Part print with two shaded views. Sizes in mm from the minimum x, y, z corner. Round coordinates to 2 decimals unless told otherwise and drop trailing zeros. Order: outer loops, then holes, each group sorted by start corner. A loop starts at its lowest first (then second) coordinate and runs counter-clockwise, first axis right, second up. Notation, with made-up numbers: M 84,37.5 L 116,37.5 A12 ccw 116,59.5 Z; hole C 54,66.5 d7. An arc over 180 degrees is marked long. One line per question, with ' | ' between items.
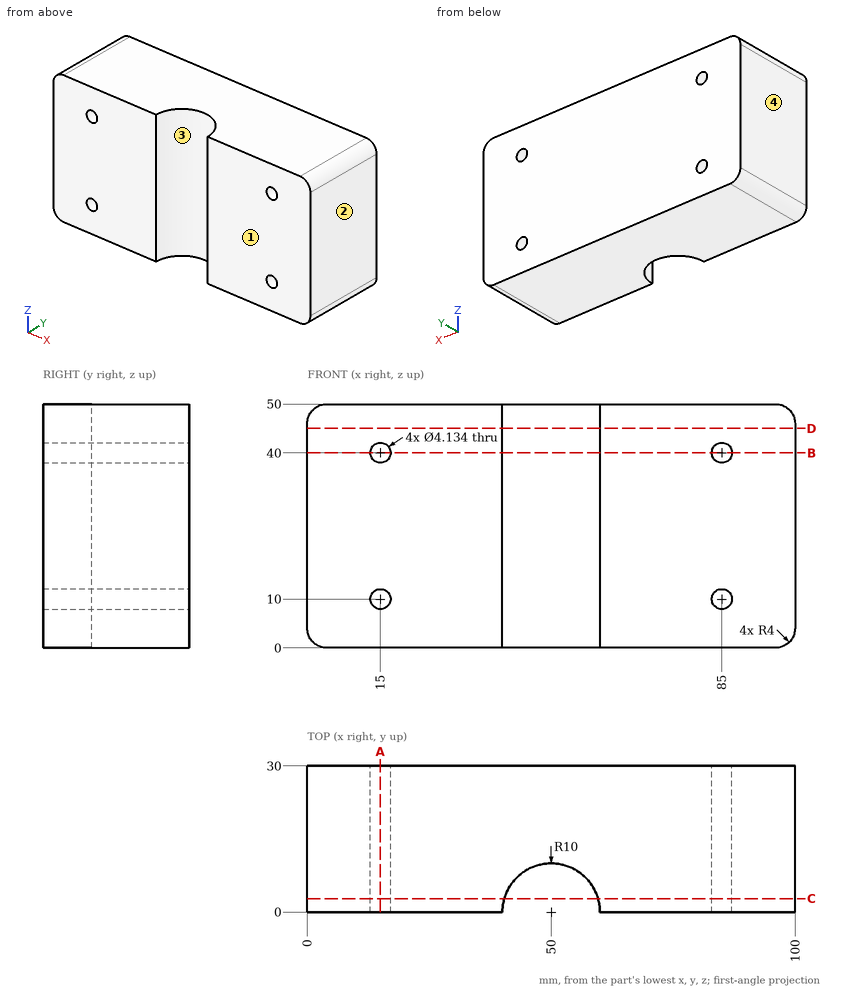
1) Saw through at D-D (z = 45). List the corners of the cut face in (x, y), plus the area to 3 significant figures.
The answers:
outline: M 0,0 L 40,0 A10 cw 60,0 L 100,0 L 100,30 L 0,30 Z | area: 2,840 mm²
2) Probe line 1 (Z direction, x = 15, y = 19.5); line 2 (X direction, y = 15, z = 10); line 3 (X direction, y = 7.5, z = 10). List the from-to ranges inside material, lowest first. Write a range as [from, to].
The answers:
line 1: z = [0, 7.93], [12.07, 37.93], [42.07, 50] | line 2: x = [0, 12.93], [17.07, 82.93], [87.07, 100] | line 3: x = [0, 12.93], [17.07, 43.39], [56.61, 82.93], [87.07, 100]
3) Saw through at B-B (z = 40). List the corners of the cut face in (x, y).
The answers:
outline: M 0,0 L 12.93,0 L 12.93,30 L 0,30 Z; M 17.07,0 L 40,0 A10 cw 60,0 L 82.93,0 L 82.93,30 L 17.07,30 Z; M 87.07,0 L 100,0 L 100,30 L 87.07,30 Z
4) Saw through at C-C (y = 2.75). List the corners of the cut face in (x, z).
The answers:
outline: M 0,4 A4 ccw 4,0 L 40.39,0 L 40.39,50 L 4,50 A4 ccw 0,46 Z; M 59.61,0 L 96,0 A4 ccw 100,4 L 100,46 A4 ccw 96,50 L 59.61,50 Z; hole C 15,10 d4.13; hole C 15,40 d4.13; hole C 85,10 d4.13; hole C 85,40 d4.13
5) Two-plate mould, pull along X, no slides. Class the marked faces 1, 2, 3 and 4: released by +X, released by -X, zero draft, split by the parting line, or undercut.
The answers:
face 1: zero draft | face 2: released by +X | face 3: undercut | face 4: released by -X
6) Saw through at A-A (x = 15). List the corners of the cut face in (y, z), plus the area to 3 significant figures.
The answers:
outline: M 0,0 L 30,0 L 30,7.93 L 0,7.93 Z; M 0,12.07 L 30,12.07 L 30,37.93 L 0,37.93 Z; M 0,42.07 L 30,42.07 L 30,50 L 0,50 Z | area: 1,250 mm²
